```python
from build123d import *

# Parameters (mm, degrees)
SKETCH1_R           = 0.875
BOSS_EXTRUDE2_DEPTH = 18
SKETCH3_R           = 4
BOSS_EXTRUDE3_DEPTH = 3
SKETCH4_R           = 0.875
BOSS_EXTRUDE4_DEPTH = 22


with BuildPart() as part:
    # Sketch1 → Boss-Extrude2 (new body)
    with BuildSketch(Plane(origin=(0, 0, 0), x_dir=(1, 0, 0), z_dir=(0, 1, 0))):
        with Locations(Location((0, 0, 0), (0, 0, 270))):
            Circle(SKETCH1_R)
    extrude(amount=BOSS_EXTRUDE2_DEPTH)

    # Sketch3 → Boss-Extrude3 (add)
    with BuildSketch(Plane(origin=(0, 18, 0), x_dir=(1, 0, 0), z_dir=(0, 1, 0))):
        with Locations(Location((0, 0, 0), (0, 0, 270))):
            Circle(SKETCH3_R)
    extrude(amount=-BOSS_EXTRUDE3_DEPTH)

    # Sketch4 → Boss-Extrude4 (add)
    with BuildSketch(Plane(origin=(0, 18, 0), x_dir=(1, 0, 0), z_dir=(0, 1, 0))):
        with Locations(Location((0, 0, 0), (0, 0, 270))):
            Circle(SKETCH4_R)
    extrude(amount=BOSS_EXTRUDE4_DEPTH)


solid = part.part
```
The model under review builds one solid part; all positions refer to its coordinate system, in mm. A direction names the side the tool comes from. Round coordinates to 2 decimals unless told otherwise and drop trailing zeros. Order: outer loops, then holes, each group sorted by start corner. A loop starts at its lowest first (then second) coordinate and runs counter-clockwise, first axis right, second up.
Item 1: Add section C-C, the plane y = 34. State the section outline as (x, z) points (3 decimals).
Working result:
outline: circle Ø1.75 at (0, 0)
Item 2: Add section B-B, the plane z = 0. State the section outline as (x, y) points (3 decimals).
Working result:
outline: (-4, 15) - (-0.875, 15) - (-0.875, 0) - (0.875, 0) - (0.875, 15) - (4, 15) - (4, 18) - (0.875, 18) - (0.875, 40) - (-0.875, 40) - (-0.875, 18) - (-4, 18) - close
Item 3: Machinability: for faces 1 (the cylindrical face through (-0.854, 7.395, -0.19)), 2 (the cylindrical face through (-0.854, 28.846, -0.19)), 3 (the flat face through (0, 0, 0)), which of the approach directions +Z, -Z, +X, -X, +Y, -Y give a long, thin tool a straight path to every point of the face, cutting with its end or side? Answer none if there is none.
Working result:
face 1: -Y
face 2: +Y
face 3: +Z, -Z, +X, -X, -Y
Item 4: Add section A-A, the plane x = 0. State the section outline as (y, z) points (3 decimals).
Working result:
outline: (0, -0.875) - (15, -0.875) - (15, -4) - (18, -4) - (18, -0.875) - (40, -0.875) - (40, 0.875) - (18, 0.875) - (18, 4) - (15, 4) - (15, 0.875) - (0, 0.875) - close
Item 5: Add section D-D, the plane x = 3.5. State the section outline as (y, z) points.
Working result:
outline: (15, -1.94) - (18, -1.94) - (18, 1.94) - (15, 1.94) - close
Item 6: For pin 1 (1 mm diameter, centred on x = 1, y = 11, fed in from +Z); pin 2 (1 mm diameter, centred on x = 1, z = -1.5, fed in from +Y); pin 3 (3 mm diameter, centred on x = 1.5, y = 33, fed in from +Z) (3 decimals); pin 4 (4 mm diameter, centred on x = -0.5, z = -1, fed in from +Y), all flat-tipped, find the tip position at first contact; note any pin that passes through.
Working result:
pin 1: stops at z = 0.72
pin 2: stops at y = 18
pin 3: stops at z = 0.875
pin 4: stops at y = 40
Item 7: To check wall thickness, follow probe 1 along Y at (x, z) = (-0.5, 2.5); probe 2 along X at (y, z) = (33.5, 0) (3 decimals); probe 3 along Z at (x, y) = (-0.5, 17). State the ranges of each line that lie inside material, in increasing order.
Working result:
probe 1: y = 15 to 18
probe 2: x = -0.875 to 0.875
probe 3: z = -3.97 to 3.97
